The listing builds one solid part. Answer for the finished solid, in the listing's coordinates (mm). Round coordinates to 2 decimals unless told otherwise and drop trailing zeros. Write each loop counter-clockwise with the first axis right and the second up, starting at its lowest first coordinate (ties: lowest second). Pieces come first, ordered by that corner, then holes. Notation, with made-up numbers: (-19, -8) -> (40, -8) arc R28 ccw to (40, 23) -> close; hole circle Ø8 at (89.5, 33). An arc over 180 degrees is marked (long way). Write each question's results on one line, items separated by ' | '. Start each with the question number.
```python
from build123d import *

# Parameters (mm, degrees)
ESBO_O1_W                               = 200
ESBO_O1_H                               = 150
RESSALTO_EXTRUS_O1_DEPTH                = 4
ESBO_O2_W                               = 35
ESBO_O2_H                               = 4
ESBO_O2_W_2                             = 4
ESBO_O2_H_2                             = 30
CORTE_EXTRUS_O1_DEPTH                   = 5
ESBO_O3_W                               = 200
ESBO_O3_H                               = 15
CORTE_EXTRUS_O2_DEPTH                   = 5
BROCA_DE_ROSQUEAR_PARA_TARRAXA_DE_M41_D = 3.3
ESBO_O5_R                               = 1.65
CORTE_EXTRUS_O3_DEPTH                   = 5


with BuildPart() as part:
    # Esboço1 → Ressalto-extrusão1 (new body)
    with BuildSketch(Plane(origin=(0, 0, 0), x_dir=(1, 0, 0), z_dir=(0, 1, 0))):
        Rectangle(ESBO_O1_W, ESBO_O1_H)
    extrude(amount=RESSALTO_EXTRUS_O1_DEPTH)

    # Esboço2 → Corte-extrusão1 (cut, through all)
    with BuildSketch(Plane(origin=(0, 4, 0), x_dir=(1, 0, 0), z_dir=(0, 1, 0))):
        with Locations((-27.5, -73)):
            Rectangle(ESBO_O2_W, ESBO_O2_H)
        with Locations((27.5, -73)):
            Rectangle(ESBO_O2_W, ESBO_O2_H)
        with Locations((82.5, -73)):
            Rectangle(ESBO_O2_W, ESBO_O2_H)
        with Locations((-82.5, -73)):
            Rectangle(ESBO_O2_W, ESBO_O2_H)
        with Locations((98, 30)):
            Rectangle(ESBO_O2_W_2, ESBO_O2_H_2)
        with Locations((98, -30)):
            Rectangle(ESBO_O2_W_2, ESBO_O2_H_2)
        with Locations((-98, 30)):
            Rectangle(ESBO_O2_W_2, ESBO_O2_H_2)
        with Locations((-98, -30)):
            Rectangle(ESBO_O2_W_2, ESBO_O2_H_2)
    extrude(amount=-CORTE_EXTRUS_O1_DEPTH, mode=Mode.SUBTRACT)

    # Esboço3 → Corte-extrusão2 (cut, through all)
    with BuildSketch(Plane(origin=(0, 4, 0), x_dir=(1, 0, 0), z_dir=(0, 1, 0))):
        with Locations((0, 67.5)):
            Rectangle(ESBO_O3_W, ESBO_O3_H)
    extrude(amount=-CORTE_EXTRUS_O2_DEPTH, mode=Mode.SUBTRACT)

    # Broca de rosquear para tarraxa de M41 (through all)
    with Locations(Plane(origin=(-85, 4, -40), x_dir=(0, 0, 1), z_dir=(0, 1, 0))):
        with Locations((0, 0), (96, 0), (96, 170), (0, 170)):
            Hole(BROCA_DE_ROSQUEAR_PARA_TARRAXA_DE_M41_D / 2)

    # Esboço5 → Corte-extrusão3 (cut, through all)
    with BuildSketch(Plane(origin=(0, 4, 0), x_dir=(1, 0, 0), z_dir=(0, 1, 0))):
        with Locations((-85, -56)):
            Circle(ESBO_O5_R)
        with BuildLine():
            Line((55, -61), (-55, -61))
            ThreePointArc((-55, -61), (-60, -56), (-55, -51))
            Line((-55, -51), (55, -51))
            ThreePointArc((55, -51), (60, -56), (55, -61))
        make_face()
    extrude(amount=-CORTE_EXTRUS_O3_DEPTH, mode=Mode.SUBTRACT)


solid = part.part
```
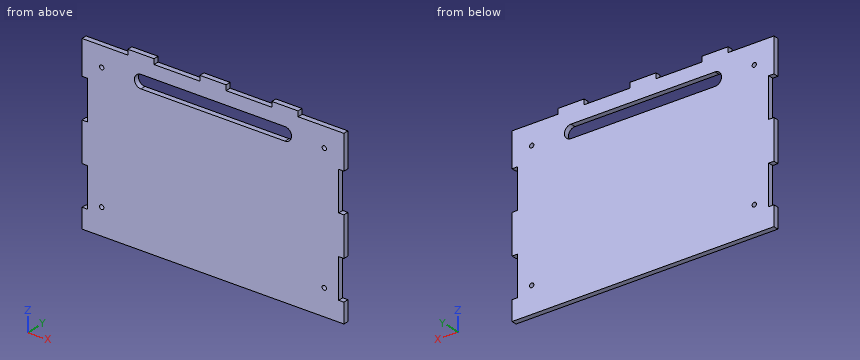
Q1. The part is cut by section A-A, the plane x = -32. Write down the section's boundary in (y, z).
Q2. The part is cut by section B-B, the plane x = -0.5. Write down the section's boundary in (y, z).
Q3. The part is cut by section D-D, the plane z = -22. Write down the section's boundary in (x, y).
Q4. Each of these flat-tipped pins is pushed along its axis until it touches: pin 1 (1.2 mm diameter, centred on x = 11, y = 2.5, fed in from +Z); pin 2 (1.2 mm diameter, centred on y = 2.5, z = 73, fed in from -X). Where does it stop, or does it pass through?
Q5. Find the intervals of material crossed by line 1 (X direction, y = 1.95, z = 56); line 2 (Z direction, x = 85, y = 1.45); line 3 (X direction, y = 2.8, z = -40), in increasing order.
Q6. The part is cut by section C-C, the plane y = 2.95. State how many separate pieces and enclosed holes the cut face has, then the cut area to 3 significant figures.
Answers follow:
1) outline: (0, -60) -> (4, -60) -> (4, 51) -> (0, 51) -> close; (0, 61) -> (4, 61) -> (4, 71) -> (0, 71) -> close
2) outline: (0, -60) -> (4, -60) -> (4, 51) -> (0, 51) -> close; (0, 61) -> (4, 61) -> (4, 75) -> (0, 75) -> close
3) outline: (-96, 0) -> (96, 0) -> (96, 4) -> (-96, 4) -> close
4) pin 1: z = 71 | pin 2: x = -65
5) line 1: -100 to -86.65, -83.35 to -60, 60 to 83.35, 86.65 to 100 | line 2: -60 to -41.65, -38.35 to 54.35, 57.65 to 71 | line 3: -96 to -86.65, -83.35 to 83.35, 86.65 to 96
6) separate pieces: 1 | enclosed holes: 5 | area: 24,700 mm^2
